```python
from build123d import *

# Parameters (mm, degrees)
F0_R     = 17.506555
F1_DEPTH = 480
F2_R     = 8.062213
F3_DEPTH = 20
F4_R     = 8.062213
F5_DEPTH = 20


with BuildPart() as f1:
    # F0 (on Top) → F1 (new body)
    with BuildSketch(Plane.XY):
        Circle(F0_R)
    extrude(amount=F1_DEPTH)

    # F2 (on Front) → F3 (join)
    with BuildSketch(Plane.XZ):
        with Locations((0, 226.747483)):
            Circle(F2_R)
    extrude(amount=F3_DEPTH)

    # F4 (on Front) → F5 (join)
    with BuildSketch(Plane.XZ):
        with Locations((0.667743, 297.020525)):
            Circle(F4_R)
    extrude(amount=F5_DEPTH)


solid = f1.part
```
Here's how the part is built. I have some questions about the finished solid (model axes, mm). A direction names the side the tool comes from. Give positions to 0.01 mm unless a question says otherwise; leave off trailing zeros. Loops run counter-clockwise (first coordinate to the right, second up) from the corner with the lowest first, then second, coordinate; pieces in that order, holes last. Notation, with made-up numbers: M 47,29 L 76,29 A23 ccw 76,40 Z; hole C -2.75,24.5 d2. An arc over 180 degrees is marked long. Use one line per item in the form item = value. Start each with the question number.
Q1. Will these pins go through, and if not, where does the flat tip stop? pin 1 Ø3 at (y, z) = (-9.5, 188) entering from +X; pin 2 Ø5 at (y, z) = (-13.5, 308) entering from -X; pin 3 Ø6 at (x, z) = (10.5, 141.5) entering from -Y.
Q2. If we section it at A-A (x = 0): Write out the boundary of the cut face in (y, z), then the cut area to 3 significant figures.
Q3. I need wall thicknesses on line 1 along Y through (x, z) = (-1, 369); line 2 along Y through (x, z) = (7.5, 416.5); line 3 along X through (y, z) = (-6.5, 265). Which ranges of each line are inside material? Lowest first, please.
Q4. If we section it at B-B (z = 250.5): Write out the boundary of the cut face in (x, y).
Q5. Which directions (+Z, -Z, +X, -X, +Y, -Y) give clear straight access to the entire face, cutting with the end or side of a thin tool? Please do faces 1 (the cylindrical face through (8.36, -18.09, 299.44)), 2 (the flat face through (0, 0, 480)).
Q6. If we section it at C-C (y = 5): Write out the boundary of the cut face in (x, z).
Taken from the geometry:
q1.pin_1 = 15.57
q1.pin_2 = -13.62
q1.pin_3 = -15.82
q2.outline = M -20,218.69 L -17.51,218.69 L -17.51,0 L 17.51,0 L 17.51,480 L -17.51,480 L -17.51,305.06 L -20,305.06 L -20,288.99 L -17.51,288.99 L -17.51,234.81 L -20,234.81 Z
q2.area = 16,900 mm^2
q3.line_1 = -17.48 to 17.48
q3.line_2 = -15.82 to 15.82
q3.line_3 = -16.26 to 16.26
q4.outline = C 0,0 d35.01
q5.face_1 = -Y
q5.face_2 = +Z, +X, -X, +Y, -Y
q6.outline = M -16.78,0 L 16.78,0 L 16.78,480 L -16.78,480 Z
